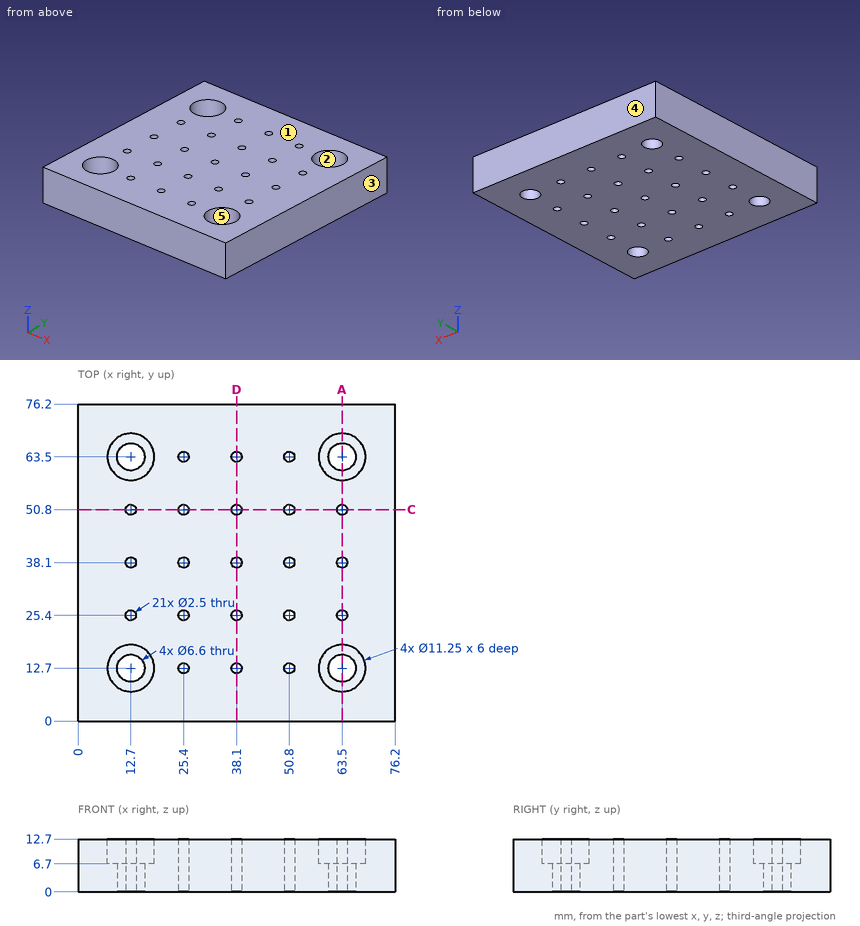
Here's the drawing with two shaded views (mm, measured from the low corner). I have some questions. A direction names the side the tool comes from. Round coordinates to 2 decimals unless told otherwise and drop trailing zeros. Order: outer loops, then holes, each group sorted by start corner. A loop starts at its lowest first (then second) coordinate and runs counter-clockwise, first axis right, second up. Notation, with made-up numbers: (-24, 37) -> (-18, 37) arc R7 ccw to (-18, 42) -> close; hole circle Ø4 at (21.25, 58.5). An arc over 180 degrees is marked (long way). Write each question's results on one line, items separated by ' | '. Start each with the question number.
Item 1: Will these pins go through, and if not, where does the flat tip stop? pin 1 (2 mm diameter, centred on x = 50.8, y = 63.5, fed in from -Z); pin 2 (3 mm diameter, centred on x = 22, y = 46, fed in from -Z); pin 3 (3.5 mm diameter, centred on x = 14, y = 62, fed in from +Z).
Item 2: Which directions (+Z, -Z, +X, -X, +Y, -Y) give clear straight access to the entire face, cutting with the end or side of a thin tool? Please do the marked faces 1 and 2.
Item 3: If we section it at A-A, the plane x = 63.5: State how many separate pieces and enclosed holes the cut face has, then the cut area to 3 significant figures.
Item 4: Thinking about a two-plate mould opening in X: for the marked faces 3, 4 and 5, which applies, +X half, -X half, draft (parallel to the pull), parting line (faces both ways), or undercut?
Item 5: If we section it at C-C, the plane y = 50.8: Write out the boundary of the cut face in (x, z).
Item 6: Please list where these lines run through material, in increasing order: L1, parallel to Y at x = 50.8, z = 9; L2, parallel to Y at x = 63.5, z = 8.75 (3 decimals); L3, parallel to Y at x = 14.5, z = 10.
Results:
1) pin 1: passes through | pin 2: stops at z = 0 | pin 3: stops at z = 6.7
2) face 1: +Z, +X, -X, +Y, -Y | face 2: +Z
3) separate pieces: 6 | enclosed holes: 0 | area: 649 mm2
4) face 3: +X half | face 4: draft | face 5: undercut
5) outline: (0, 0) -> (11.45, 0) -> (11.45, 12.7) -> (0, 12.7) -> close; (13.95, 0) -> (24.15, 0) -> (24.15, 12.7) -> (13.95, 12.7) -> close; (26.65, 0) -> (36.85, 0) -> (36.85, 12.7) -> (26.65, 12.7) -> close; (39.35, 0) -> (49.55, 0) -> (49.55, 12.7) -> (39.35, 12.7) -> close; (52.05, 0) -> (62.25, 0) -> (62.25, 12.7) -> (52.05, 12.7) -> close; (64.75, 0) -> (76.2, 0) -> (76.2, 12.7) -> (64.75, 12.7) -> close
6) L1: y = 0 to 11.45, 13.95 to 24.15, 26.65 to 36.85, 39.35 to 49.55, 52.05 to 62.25, 64.75 to 76.2 | L2: y = 0 to 7.075, 18.325 to 24.15, 26.65 to 36.85, 39.35 to 49.55, 52.05 to 57.875, 69.125 to 76.2 | L3: y = 0 to 7.37, 18.03 to 58.17, 68.83 to 76.2
